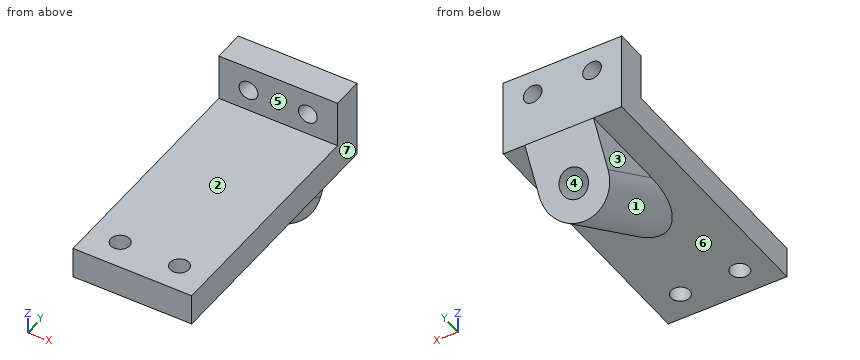
```python
from build123d import *

# Parameters (mm, degrees)
SKETCH1_W           = 76
SKETCH1_H           = 50
SKETCH1_R           = 6
BOSS_EXTRUDE1_DEPTH = 20
SKETCH2_W           = 76
SKETCH2_H           = 20
BOSS_EXTRUDE2_DEPTH = 150
SKETCH3_R           = 6
CUT_EXTRUDE1_DEPTH  = 150
BOSS_EXTRUDE3_REACH = 186.259
SKETCH5_R           = 9


with BuildPart() as part:
    # Sketch1 → Boss-Extrude1 (new body)
    with BuildSketch(Plane(origin=(0, 0, 0), x_dir=(1, 0, 0), z_dir=(0, 1, 0))):
        Rectangle(SKETCH1_W, SKETCH1_H)
        with Locations(Location((-19, -9, 0), (0, 0, 270))):
            Circle(SKETCH1_R, mode=Mode.SUBTRACT)
        with Locations(Location((19, -9, 0), (0, 0, 90))):
            Circle(SKETCH1_R, mode=Mode.SUBTRACT)
    extrude(amount=BOSS_EXTRUDE1_DEPTH)

    # Sketch2 → Boss-Extrude2 (add)
    with BuildSketch(Plane.XZ):
        with Locations((0, -15)):
            Rectangle(SKETCH2_W, SKETCH2_H)
    extrude(amount=BOSS_EXTRUDE2_DEPTH)

    # Sketch3 → Cut-Extrude1 (cut)
    with BuildSketch(Plane(origin=(0, 0, -25), x_dir=(-1, 0, 0), z_dir=(0, 0, -1))):
        with Locations((-19, -132)):
            Circle(SKETCH3_R)
        with Locations((19, -132)):
            Circle(SKETCH3_R)
    extrude(amount=-CUT_EXTRUDE1_DEPTH, mode=Mode.SUBTRACT)

    # Sketch5 → Boss-Extrude3 (add, up to next)
    with BuildSketch(Plane(origin=(0, 25.825317547, -14.910254038), x_dir=(1, 0, 0), z_dir=(0, -0.8660254037844399, 0.4999999999999977)), mode=Mode.PRIVATE) as boss_extrude3_sk1:
        with BuildLine():
            Line((-19.931985631, -11.650635095), (24.068014369, -11.650635095))
            Line((24.068014369, -11.650635095), (24.068014369, -41.650635095))
            ThreePointArc((24.068014369, -41.650635095), (2.068014369, -63.650635095), (-19.931985631, -41.650635095))
            Line((-19.931985631, -41.650635095), (-19.931985631, -11.650635095))
        make_face()
        with Locations(Location((2.068014369, -41.650635095, 0), (0, 0, 90))):
            Circle(SKETCH5_R, mode=Mode.SUBTRACT)
    boss_extrude3_tool1 = extrude(boss_extrude3_sk1.sketch, amount=BOSS_EXTRUDE3_REACH, mode=Mode.PRIVATE) - part.part
    add(boss_extrude3_tool1.solids().sort_by_distance((-19.25081, 12.5, -37.990381))[0])


solid = part.part
```
Design review of the part built by this model. Coordinates are the model's own, in mm. Face numbers are marked on the shaded views. A direction names the side the tool comes from. Give positions to 0.01 mm unless a question says otherwise; leave off trailing zeros. Write each loop counter-clockwise with the first axis right and the second up, starting at its lowest first coordinate (ties: lowest second). Pieces come first, ordered by that corner, then holes.
(1) Mouldability with a two-part tool opening along X and no side actions: class the marked faces 1, 2, 3 and 4 as +X half, -X half, draft (parallel to the pull), parting line (faces both ways), or undercut.
Checked values:
face 1: parting line
face 2: draft
face 3: -X half
face 4: undercut
(2) Add section A-A (y = -132). Give the boundary of the cut face in (x, z).
Checked values:
outline: (-38, -25) - (-25, -25) - (-25, -5) - (-38, -5) - close; (-13, -25) - (13, -25) - (13, -5) - (-13, -5) - close; (25, -25) - (38, -25) - (38, -5) - (25, -5) - close
(3) Clearance check with flat-ended pins moving along their axes: pin 1 Ø23 at (x, y) = (-13, -103.5) entering from +Z; pin 2 Ø10 at (y, z) = (-10, -38.5) entering from +X; pin 3 Ø9 at (x, z) = (2, 2.5) entering from -Y. State where each tip first meets the part, or that it passes through.
Checked values:
pin 1: stops at z = -5
pin 2: stops at x = 24.07
pin 3: stops at y = 0
(4) Add section C-C (x = -27.5). Give the boundary of the cut face in (y, z), and give its area (3 significant figures).
Checked values:
outline: (-150, -25) - (20, -25) - (20, 25) - (0, 25) - (0, -5) - (-150, -5) - close
area: 4,000 mm2
(5) Add section D-D (z = -10). Give the boundary of the cut face in (x, y).
Checked values:
outline: (-38, -150) - (38, -150) - (38, 20) - (-38, 20) - close; hole circle Ø12 at (-19, -132); hole circle Ø12 at (19, -132)
(6) Add section B-B (z = 9). Give the boundary of the cut face in (x, y), and give its area (3 significant figures).
Checked values:
outline: (-38, 0) - (-25, 0) - (-25, 20) - (-38, 20) - close; (-13, 0) - (13, 0) - (13, 20) - (-13, 20) - close; (25, 0) - (38, 0) - (38, 20) - (25, 20) - close
area: 1,040 mm2
(7) Tool access review of the marked faces 5, 6 and 7: name each direction out of +Z, -Z, +X, -X, +Y, -Y from which nothing blocks a thin tool from reaching the whole face with its end or side.
Checked values:
face 5: +Z, +X, -X, -Y
face 6: -Z, -Y
face 7: +Z, -Z, +X, +Y, -Y
(8) Wall thickness on line 1 along X through (y, z) = (15, 9); line 2 along Y through (x, z) = (-19, -14.5); line 3 along Y through (x, z) = (-31.5, 1): over which ranges is each line inside the solid? List them lowest first.
Checked values:
line 1: x = -38 to -25, -13 to 13, 25 to 38
line 2: y = -150 to -138, -126 to 20
line 3: y = 0 to 20
